from build123d import *

# Parameters (mm, degrees)
F0_W     = 16
F0_H     = 29
F0_W_2   = 13
F0_H_2   = 17
F1_DEPTH = 2
F2_DEPTH = 6
F3_DEPTH = 3


with BuildPart() as f1:
    # F0 (on Top) → F1 (new body)
    with BuildSketch(Plane.XY):
        Rectangle(F0_W, F0_H)
        with BuildLine():
            ThreePointArc((7.2759241834, -7.75), (6.6169144411, -9.3409902577), (5.0259241834, -10))
            Line((5.0259241834, -10), (-5.0259241834, -10))
            Line((-5.0259241834, -10), (-5.0259241834, -9.9706540408))
            ThreePointArc((-5.0259241834, -9.9706540408), (-7.2465782242, -7.75), (-5.0259241834, -5.5293459592))
            Line((-5.0259241834, -5.5293459592), (-5.0259241834, -5.5))
            Line((-5.0259241834, -5.5), (5.0259241834, -5.5))
            ThreePointArc((5.0259241834, -5.5), (6.6169144411, -6.1590097423), (7.2759241834, -7.75))
        make_face(mode=Mode.SUBTRACT)
        with Locations((0, 4.5)):
            Rectangle(F0_W_2, F0_H_2, mode=Mode.SUBTRACT)
    extrude(amount=F1_DEPTH)

    # F0 (on Top) → F2 (join)
    with BuildSketch(Plane.XY):
        with BuildLine():
            Line((-5.0259241834, -5.5293459592), (-5.0259241834, -9.9706540408))
            ThreePointArc((-5.0259241834, -9.9706540408), (-3.4556846525, -9.3202395309), (-2.8052701426, -7.75))
            ThreePointArc((-2.8052701426, -7.75), (-3.4556846525, -6.1797604691), (-5.0259241834, -5.5293459592))
        make_face()
        with BuildLine():
            ThreePointArc((-5.0259241834, -5.5293459592), (-7.2465782242, -7.75), (-5.0259241834, -9.9706540408))
            Line((-5.0259241834, -9.9706540408), (-5.0259241834, -5.5293459592))
        make_face()
        with BuildLine():
            ThreePointArc((5.0259241834, -5.5), (2.7759241834, -7.75), (5.0259241834, -10))
            Line((5.0259241834, -10), (5.0259241834, -5.5))
        make_face()
        with BuildLine():
            Line((5.0259241834, -5.5), (5.0259241834, -10))
            ThreePointArc((5.0259241834, -10), (6.6169144411, -9.3409902577), (7.2759241834, -7.75))
            ThreePointArc((7.2759241834, -7.75), (6.6169144411, -6.1590097423), (5.0259241834, -5.5))
        make_face()
        with BuildLine():
            Line((-5.0259241834, -10), (5.0259241834, -10))
            ThreePointArc((5.0259241834, -10), (2.7759241834, -7.75), (5.0259241834, -5.5))
            Line((5.0259241834, -5.5), (-5.0259241834, -5.5))
            Line((-5.0259241834, -5.5), (-5.0259241834, -5.5293459592))
            ThreePointArc((-5.0259241834, -5.5293459592), (-3.4556846525, -6.1797604691), (-2.8052701426, -7.75))
            ThreePointArc((-2.8052701426, -7.75), (-3.4556846525, -9.3202395309), (-5.0259241834, -9.9706540408))
            Line((-5.0259241834, -9.9706540408), (-5.0259241834, -10))
        make_face()
    extrude(amount=F2_DEPTH)

    # F0 (on Top) → F3 (join)
    with BuildSketch(Plane.XY):
        with Locations((0, 4.5)):
            Rectangle(F0_W_2, F0_H_2)
    extrude(amount=F3_DEPTH)


solid = f1.part
Model file for the job. Use its own axes, mm. A direction names the side the tool comes from. Round coordinates to 2 decimals unless told otherwise and drop trailing zeros. Order: outer loops, then holes, each group sorted by start corner. A loop starts at its lowest first (then second) coordinate and runs counter-clockwise, first axis right, second up.
(1) Pin check, flat tips, straight feed: pin 1 (1.2 mm diameter, centred on x = 2, z = 4, fed in from -Y); pin 2 (2 mm diameter, centred on x = 1, z = 4.5, fed in from +Y). Stop position of each tip, or through.
(2) 3-axis set-ups, long thin cutter, end or side, ignore diameter. For faces 1 (the face through (6.5, 4.4, 2.5)), 2 (the face through (0, -10, 4)), 3 (the face through (-7.246, -7.701, 3.972)), 4 (the face through (0, -5.5, 4)), 5 (the face through (-6.5, 4.4, 2.5)): which of +Z, -Z, +X, -X, +Y, -Y reach the whole face in a straight line?
(3) Drill centre lines: line 1 (Y direction, x = -2.75, z = 2.3); line 2 (Z direction, x = -3, y = 5); line 3 (Y direction, x = -0.5, z = 5.5). Where is each one in solid material? Low to high.
(4) Pull direction Y, two halves, no side cores. Call faces 6 (the face through (8, 0, 1)), 7 (the face through (0, 14.5, 1)), 8 (the face through (-0.1, -4, 2.5)): released by +Y, released by -Y, zero draft, split by the parting line, or undercut.
(5) Band-saw the part on B-B (x = 5.75). List the corners of the cut face in (y, z).
(6) Band-saw the part on C-C (y = 6.25). List the corners of the cut face in (x, z).
(7) Band-saw the part on D-D (y = -7). List the corners of the cut face in (x, z), then the cut area to 3 significant figures.
Verdict:
1. pin 1: stops at y = -10
1. pin 2: stops at y = -5.5
2. face 1: +Z, +X, +Y
2. face 2: +Z, +X, -X, -Y
2. face 3: +Z, -X
2. face 4: +Z, +X, -X
2. face 5: +Z, -X, +Y
3. line 1: y = -10 to -5.5, -4 to 13
3. line 2: z = 0 to 3
3. line 3: y = -10 to -5.5
4. face 6: zero draft
4. face 7: released by +Y
4. face 8: undercut
5. outline: (-14.5, 0) - (14.5, 0) - (14.5, 2) - (13, 2) - (13, 3) - (-4, 3) - (-4, 2) - (-5.62, 2) - (-5.62, 6) - (-9.88, 6) - (-9.88, 2) - (-14.5, 2) - close
6. outline: (-8, 0) - (8, 0) - (8, 2) - (6.5, 2) - (6.5, 3) - (-6.5, 3) - (-6.5, 2) - (-8, 2) - close
7. outline: (-8, 0) - (8, 0) - (8, 2) - (7.15, 2) - (7.15, 6) - (-7.12, 6) - (-7.12, 2) - (-8, 2) - close
7. area: 89.1 mm2
